from build123d import *

# Parameters (mm, degrees)
F0_W     = 18.8587028533
F0_H     = 9.4020338729
F1_DEPTH = 12.5
F2_R     = 5.1767234365
F3_DEPTH = 25


with BuildPart() as f1:
    # F0 (on Front) → F1 (new body, symmetric)
    with BuildSketch(Plane.XZ):
        Rectangle(F0_W, F0_H)
    extrude(amount=F1_DEPTH, both=True)

    # F2 (on face) → F3 (cut)
    with BuildSketch(Plane.XY.offset(4.7010169365)):
        Circle(F2_R)
    extrude(amount=-F3_DEPTH, mode=Mode.SUBTRACT)


solid = f1.part
Here's how the part is built. I have some questions about the finished solid (model axes, mm). Round coordinates to 2 decimals unless told otherwise and drop trailing zeros. Order: outer loops, then holes, each group sorted by start corner. A loop starts at its lowest first (then second) coordinate and runs counter-clockwise, first axis right, second up. Notation, with made-up numbers: M 13,-23.5 L 68,-23.5 A17 cw 68,5.5 Z; hole C -22.75,30 d5. An arc over 180 degrees is marked long. Return JSON: item names as keys, results as strings. Group by question number.
1. If we section it at A-A on y = 0: List the corners of the cut face in (x, z) for me.
2. If we section it at B-B on x = 0: List the corners of the cut face in (y, z) for me, then the cut area to 3 significant figures.
3. If we mould it in two halves opening along Y, with no side actions, what happens to faces 1 (the face through (2.783, 4.365, 0.066)), 2 (the face through (-9.429, 0, 0)), 3 (the face through (0, 12.5, 0))? For each: pulls with the +Y half, pulls with the -Y half, needs draft (parallel to the pull), parting line crosses it, or undercut.
4. I'm going to push a flat-ended pin straight in: pin 1 Ø6 at (x, y) = (0, 0) entering from +Z. Where does the tip first touch, or does it pass through?
5. Please list where these lines run through material, in increasing order: probe 1 along Y at (x, z) = (0, -1.75); probe 2 along X at (y, z) = (2, 0.25); probe 3 along Y at (x, z) = (2.75, -3).
Reply:
{
 "1": {"outline": "M -9.43,-4.7 L -5.18,-4.7 L -5.18,4.7 L -9.43,4.7 Z; M 5.18,-4.7 L 9.43,-4.7 L 9.43,4.7 L 5.18,4.7 Z"},
 "2": {"outline": "M -12.5,-4.7 L -5.18,-4.7 L -5.18,4.7 L -12.5,4.7 Z; M 5.18,-4.7 L 12.5,-4.7 L 12.5,4.7 L 5.18,4.7 Z", "area": "138 mm^2"},
 "3": {"face 1": "undercut", "face 2": "needs draft", "face 3": "pulls with the +Y half"},
 "4": {"pin 1": "through"},
 "5": {"probe 1": "-12.5 to -5.18, 5.18 to 12.5", "probe 2": "-9.43 to -4.77, 4.77 to 9.43", "probe 3": "-12.5 to -4.39, 4.39 to 12.5"}
}
